from build123d import *

# Parameters (mm, degrees)
SKETCH1_W               = 23
SKETCH1_H               = 15
BOSS_EXTRUDE1_DEPTH     = 30
SKETCH2_W               = 11
SKETCH2_H               = 15
CUT_EXTRUDE1_DEPTH      = 25
CUT_EXTRUDE2_DEPTH      = 41.669398815
CUT_EXTRUDE2_DEPTH_BACK = 41.669398815
SKETCH3_R               = 1.7
CHAMFER1_SIZE           = 2.5
CHAMFER1_SIZE_2         = 14.178204549
SKETCH4_R               = 2.2
CUT_EXTRUDE3_DEPTH      = 10
CUT_EXTRUDE4_DEPTH      = 2
SKETCH6_R               = 3.25
CUT_EXTRUDE5_DEPTH      = 2.5
CUT_EXTRUDE6_DEPTH      = 3.8
CHAMFER3_SIZE           = 1


with BuildPart() as part:
    # Sketch1 → Boss-Extrude1 (new body)
    with BuildSketch(Plane(origin=(0, 0, 0), x_dir=(0, 0, -1), z_dir=(1, 0, 0))):
        with Locations((11.5, 7.5)):
            Rectangle(SKETCH1_W, SKETCH1_H)
    extrude(amount=BOSS_EXTRUDE1_DEPTH)

    # Sketch2 → Cut-Extrude1 (cut)
    with BuildSketch(Plane(origin=(30, 0, 0), x_dir=(0, 0, -1), z_dir=(1, 0, 0))):
        with Locations((11.5, 7.5)):
            Rectangle(SKETCH2_W, SKETCH2_H)
    extrude(amount=-CUT_EXTRUDE1_DEPTH, mode=Mode.SUBTRACT)

    # Sketch3 → Cut-Extrude2 (cut, two sides: drawn at the far end of the back side and taken through both)
    with BuildSketch(Plane(origin=(0, 0, -23), x_dir=(-1, 0, 0), z_dir=(0, 0, -1)).offset(-CUT_EXTRUDE2_DEPTH_BACK)):
        with Locations(Location((-26, 9.5, 0), (0, 0, 90))):
            Circle(SKETCH3_R)
    extrude(amount=CUT_EXTRUDE2_DEPTH + CUT_EXTRUDE2_DEPTH_BACK, mode=Mode.SUBTRACT)

    # Chamfer1
    # the kernel refuses this chamfer: 14.178204549, 2.5 mm, written as the material it takes off along each edge
    with BuildSketch(Plane(origin=(0, 15, -59.842614584), x_dir=(-0.21013876076743537, -0.9776715712462578, 0), z_dir=(0, 0, 1))) as chamfer1_piece_1:
        Polygon((CHAMFER1_SIZE * 0.977671571246, CHAMFER1_SIZE * 0.210138760767), (-CHAMFER1_SIZE_2 * 0.210138760768, CHAMFER1_SIZE_2 * 0.977671571249), (0, 0), align=None)
    extrude(amount=96.685229169, mode=Mode.SUBTRACT)

    # Sketch4 → Cut-Extrude3 (cut)
    with BuildSketch(Plane.ZY):
        with Locations((-11.5, 6.25)):
            Circle(SKETCH4_R)
    extrude(amount=-CUT_EXTRUDE3_DEPTH, mode=Mode.SUBTRACT)

    # Sketch5 → Cut-Extrude4 (cut)
    with BuildSketch(Plane(origin=(5, 0, 0), x_dir=(0, 0, -1), z_dir=(1, 0, 0))):
        Polygon((7.9, 8.328460969), (7.9, 4.171539031), (11.5, 2.093078062), (15.1, 4.171539031), (15.1, 8.328460969), (11.5, 10.406921938), align=None)
    extrude(amount=-CUT_EXTRUDE4_DEPTH, mode=Mode.SUBTRACT)

    # Sketch6 → Cut-Extrude5 (cut)
    with BuildSketch(Plane(origin=(0, 0, -23), x_dir=(-1, 0, 0), z_dir=(0, 0, -1))):
        with Locations((-26, 9.5)):
            Circle(SKETCH6_R)
    extrude(amount=-CUT_EXTRUDE5_DEPTH, mode=Mode.SUBTRACT)

    # Sketch7 → Cut-Extrude6 (cut)
    with BuildSketch(Plane.XY):
        Polygon((23.1, 11.174315781), (23.1, 7.825684219), (26, 6.151368439), (28.9, 7.825684219), (28.9, 11.174315781), (26, 12.848631561), align=None)
    extrude(amount=-CUT_EXTRUDE6_DEPTH, mode=Mode.SUBTRACT)

    # Chamfer3
    chamfer3_edges = [part.edges().sort_by_distance(p)[0] for p in [
        (5, 6.690817452, -17),
        (5, 6.690817452, -6),
    ]]
    chamfer(chamfer3_edges, length=CHAMFER3_SIZE)


solid = part.part
CAD build for the part. Positions are in the model's coordinates, mm. A direction names the side the tool comes from. Give positions to 0.01 mm unless a question says otherwise; leave off trailing zeros. Write each loop counter-clockwise with the first axis right and the second up, starting at its lowest first coordinate (ties: lowest second). Pieces come first, ordered by that corner, then holes. Notation, with made-up numbers: M 75.25,18.25 L 115.25,18.25 A26 ccw 115.25,57.25 Z; hole C 5.25,32 d1. An arc over 180 degrees is marked long. Put each result on its own line as item: value. Start each with the question number.
(1) Probe L1, parallel to Z at x = 28, y = 3; L2, parallel to Z at x = 4, y = 4.75; L3, parallel to Y at x = 1.4, z = -11.5. List the from-to ranges inside material, lowest first.
(2) Band-saw the part on C-C, the plane y = 9.5. Give the number of separate pieces and of enclosed holes in the cut face, and give its area (3 significant figures).
(3) Flat gauge pins, fed straight in: pin 1 Ø4.5 at (y, z) = (8, -13) entering from +X; pin 2 Ø2.5 at (x, y) = (26, 9.5) entering from -Z; pin 3 Ø4 at (x, y) = (26, 9.5) entering from +Z; pin 4 Ø6 at (y, z) = (6, -12) entering from +X. Where does each tip first touch, or does it go through?
(4) Band-saw the part on D-D, the plane z = -13.25. Write the cut outline in (x, y), and give its area (3 significant figures).
(5) Band-saw the part on A-A, the plane z = -17.5. Write the cut outline in (x, y), and give its area (3 significant figures).
(6) Mould opens along Z. For faces 1 (the face through (24.7, 8.1, -3.8)), 2 (the face through (23.1, 10, -2)), 3 (the face through (4, 6, -7.9)) say: +Z half, -Z half, draft (parallel to the pull), parting line (faces both ways), or undercut.
(7) Band-saw the part on B-B, the plane x = 16. Write the cut outline in (y, z).
(8) Which spindle directions (+Z, -Z, +X, -X, +Y, -Y) get a long thin tool onto all of the face, cutting with end or side? Do faces 4 (the face through (24.53, 7, -1.87)), 5 (the face through (4.01, 3.15, -9.67)), 6 (the face through (26.423, 12.722, -21.768)), 7 (the face through (1.479, 8.105, -10.317)), 8 (the face through (5.5, 6.7, -6.5)). Say none if no direction does.
Response values:
1. L1: z = -23 to -17, -6 to 0
1. L2: z = -23 to -15.1, -7.9 to 0
1. L3: y = 0 to 4.05, 8.45 to 12.75
2. separate pieces: 3
2. enclosed holes: 0
2. area: 352 mm2
3. pin 1: stops at x = 5
3. pin 2: passes through
3. pin 3: stops at z = -3.8
3. pin 4: stops at x = 3
4. outline: M 0,0 L 5,0 L 5,3.1 L 3,3.1 L 3,4.92 L 0,4.92 Z; M 0,7.58 L 3,7.58 L 3,9.4 L 5,9.4 L 5,13.38 L 0,12.5 Z
4. area: 44.1 mm2
5. outline: M 0,0 L 30,0 L 30,15 L 14.18,15 L 0,12.5 Z; hole C 26,9.5 d3.4
5. area: 423 mm2
6. face 1: +Z half
6. face 2: draft
6. face 3: undercut
7. outline: M 0,-23 L 15,-23 L 15,-17 L 0,-17 Z; M 0,-6 L 15,-6 L 15,0 L 0,0 Z
8. face 4: +Z
8. face 5: +X
8. face 6: -Z
8. face 7: +X, -X
8. face 8: +X, +Y, -Y
